Autodesk Inventor part; units mm, degrees
ref_plane "YZ Plane" through (0, 0, 0) normal (1, 0, 0) x (0, 1, 0)
ref_plane "XZ Plane" through (0, 0, 0) normal (0, 1, 0) x (-1, 0, 0)
ref_plane "XY Plane" through (0, 0, 0) normal (0, 0, 1) x (1, 0, 0)
sketch "Skizze1" plane through (0, 0, 0) normal (0, 1, 0) x (-1, 0, 0)
  circle A0 centre (0, 0) radius 10
  circle A1 centre (0, 0) radius 250
  circle A2 centre (0, 0) radius 200
  circle A3 centre (0, 0) radius 25
  line L0 (10, 0) -> (10, -249.7999)
  line L1 (-10, 0) -> (-10, -249.7999)
  line L2 (0, 10) -> (249.7999, 10)
  line L3 (0, -10) -> (249.7999, -10)
  line L4 (10, 0) -> (10, 249.7999)
  line L5 (-10, 0) -> (-10, 249.7999)
  line L6 (0, 10) -> (-199.7498, 10)
  line L7 (0, -10) -> (-199.7498, -10)
  point P0 (-10, -199.7498)
  point P1 (-22.9129, -10)
  point P2 (-10, -22.9129)
  point P3 (10, -199.7498)
  point P4 (10, -22.9129)
  point P5 (22.9129, -10)
  point P6 (199.7498, -10)
  point P7 (-10, 199.7498)
  point P8 (-10, 22.9129)
  point P9 (-22.9129, 10)
  point P10 (22.9129, 10)
  point P11 (10, 22.9129)
  point P12 (10, 199.7498)
  point P13 (199.7498, 10)
  dimension "d0" = 20
  dimension "d1" = 500
  dimension "d2" = 400
  dimension "d3" = 50
extrude "Extrusion1" add sketch "Skizze1" along normal blind 10 contours L0 L3 A0 | L4 L2 A3 L3 L0 | A0 L2 L4 | L6 L5 A3 L4 L2 | A0 L5 L6 | L7 L1 A0 | L3 L0 A3 L1 L7 | L3 A3 L0 | L4 A3 L2 | L1 L7 A3 L6 L5 | L6 A3 L5 | L1 A3 L7 | L0 A2 L1 A3 | A3 L2 A2 L3 | A3 L5 A2 L4 | A3 L7 A2 L6 | L0 A1 L1 A2 | A2 L3 A1 L0 | A2 L2 A1 L3 | A2 L4 A1 L2 | A2 L5 A1 L4 | A2 L1 A1 L5
sketch "Skizze2" plane through (0, 10, 0) normal (0, 1, 0) x (1, 0, 0)
  line L0 (0, 22.9129) -> (0, 232.9129)
  circle A0 centre (0, 232.9129) radius 5
  circle A1 centre (0, 22.9129) radius 5
  line L1 (5, 232.9129) -> (5, 22.9129)
  line L2 (-5, 232.9129) -> (-5, 22.9129)
  line L3 (22.9129, 0) -> (232.9129, 0)
  circle A2 centre (232.9129, 0) radius 5
  circle A3 centre (22.9129, 0) radius 5
  line L4 (232.9129, -5) -> (22.9129, -5)
  line L5 (232.9129, 5) -> (22.9129, 5)
  line L6 (0, -22.9129) -> (0, -232.9129)
  circle A4 centre (0, -232.9129) radius 5
  circle A5 centre (0, -22.9129) radius 5
  line L7 (-5, -232.9129) -> (-5, -22.9129)
  line L8 (5, -232.9129) -> (5, -22.9129)
  line L9 (-22.9129, 0) -> (-232.9129, 0)
  circle A6 centre (-232.9129, 0) radius 5
  circle A7 centre (-22.9129, 0) radius 5
  line L10 (-232.9129, 5) -> (-22.9129, 5)
  line L11 (-232.9129, -5) -> (-22.9129, -5)
  point P0 (0, 0)
  point P1 (0, 0)
  point P2 (0, 0)
  point P3 (0, 0)
  dimension "nutlange" = 210
  dimension "radius" = 10
  dimension "d10" = 10
  dimension "d13" = 360
extrude "Extrusion2" cut sketch "Skizze2" against normal blind 5
properties part number "Seitenscheibe" material "PVC, hart"
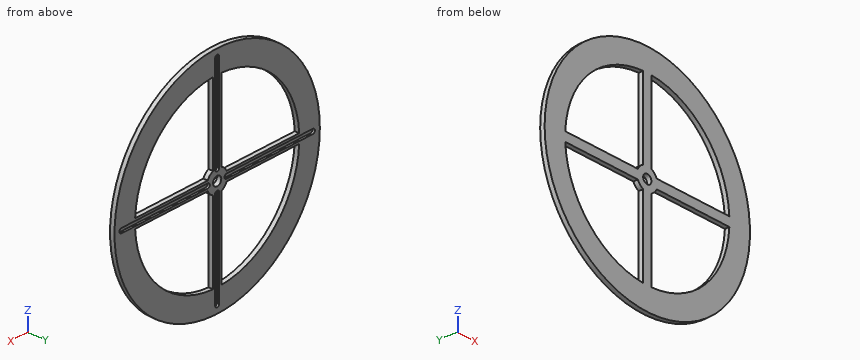
The listing builds one solid part. Answer for the finished solid, in the listing's coordinates (mm). Give positions to 0.01 mm unless a question says otherwise; leave off trailing zeros. Loops run counter-clockwise (first coordinate to the right, second up) from the corner with the lowest first, then second, coordinate; pieces in that order, holes last. Notation, with made-up numbers: (35, 88) - (85, 88) arc R31 ccw to (85, 114) - close; hole circle Ø2 at (5, -6). An arc over 180 degrees is marked (long way). Return JSON: item names as keys, results as strings. Group by question number.
1. Find section C-C (y = 8.5). State how many separate pieces and enclosed holes the cut face has, then the cut area to 3 significant figures.
2. Given pin 1 Ø4 at (x, y) = (-166.5, 8.5) entering from -Z; pin 2 Ø1.5 at (y, z) = (7, -119) entering from +X; pin 3 Ø2.5 at (x, y) = (90.5, 7.5) entering from -Z, each flat-ended and moving along its own axis, determine where each tip first touches the part or whether it passes through.
3. Find section B-B (z = -116). Write down the section's boundary in (x, y).
4. Straight lines are drawn through the part: line 1 (X direction, y = 6, z = 0); line 2 (Z direction, x = 28, y = 6.5). For each, find the intervals that lie inside material, in ascending order. Write a range as [from, to].
5. Find section A-A (x = -54). Write down the section's boundary in (y, z), then the cut area to 3 significant figures.
Verdict:
{
 "1": {"separate pieces": "1", "enclosed holes": "9", "area": "77,700 mm^2"},
 "2": {"pin 1": "stops at z = -188.25", "pin 2": "stops at x = 220.27", "pin 3": "stops at z = -233.53"},
 "3": {"outline": "(-221.46, 0) - (-162.92, 0) - (-162.92, 10) - (-221.46, 10) - close; (-10, 0) - (10, 0) - (10, 10) - (5, 10) - (5, 5) - (-5, 5) - (-5, 10) - (-10, 10) - close; (162.92, 0) - (221.46, 0) - (221.46, 10) - (162.92, 10) - close"},
 "4": {"line 1": "x = [-250, -237.91], [-17.91, -10], [10, 17.91], [237.91, 250]", "line 2": "z = [-248.43, -198.03], [-10, -5], [5, 10], [198.03, 248.43]"},
 "5": {"outline": "(0, -244.1) - (10, -244.1) - (10, -192.57) - (0, -192.57) - close; (0, -10) - (10, -10) - (10, -5) - (5, -5) - (5, 5) - (10, 5) - (10, 10) - (0, 10) - close; (0, 192.57) - (10, 192.57) - (10, 244.1) - (0, 244.1) - close", "area": "1,180 mm^2"}
}
